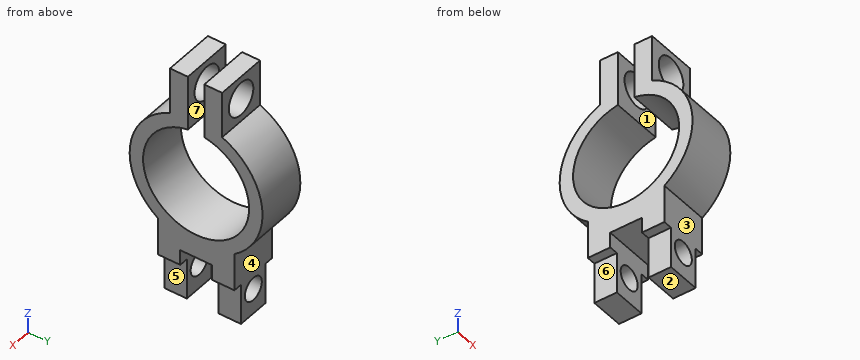
```python
from build123d import *

# Parameters (mm, degrees)
PAD_DEPTH       = 10
POCKET_DEPTH    = 10
SKETCH004_R     = 3.25
POCKET002_DEPTH = 15
SKETCH005_R     = 2.25
POCKET003_DEPTH = 15
SKETCH006_W     = 8
SKETCH006_H     = 1.75
POCKET004_DEPTH = 15


with BuildPart() as part:
    # Sketch → Pad (new body)
    with BuildSketch(Plane.YZ):
        with BuildLine():
            ThreePointArc((-1.6, 10.250884), (0, -10.375), (1.6, 10.250884))
            Line((1.6, 20.997843), (1.6, 10.250884))
            Line((1.6, 20.997843), (5.1, 20.997843))
            Line((5.1, 20.997843), (5.1, 11.957843))
            ThreePointArc((7.5, -10.61838), (12.92716, 1.374242), (5.1, 11.957843))
            Line((7.5, -25.99838), (7.5, -10.61838))
            Line((-7.5, -25.99838), (7.5, -25.99838))
            Line((-7.5, -25.99838), (-7.5, -10.61838))
            ThreePointArc((-5.1, 11.957843), (-12.92716, 1.374242), (-7.5, -10.61838))
            Line((-5.1, 20.997843), (-5.1, 11.957843))
            Line((-1.6, 20.997843), (-5.1, 20.997843))
            Line((-1.6, 20.997843), (-1.6, 10.250884))
        make_face()
    extrude(amount=PAD_DEPTH)

    # Sketch003 → Pocket (cut)
    with BuildSketch(Plane(origin=(0, 0, 0), x_dir=(0, 1, 0), z_dir=(-1, 0, 0))):
        Polygon((0, 25.99838), (-3.1, 25.99838), (-3.1, 14.99838), (0, 14.99838), (3.1, 14.99838), (3.1, 25.99838), align=None)
    extrude(amount=-POCKET_DEPTH, mode=Mode.SUBTRACT)

    # Sketch004 (on Face9 of Pocket) → Pocket002 (cut)
    with BuildSketch(Plane.ZX.offset(5.1)):
        with Locations((16.507843, 5)):
            Circle(SKETCH004_R)
    extrude(amount=-POCKET002_DEPTH, mode=Mode.SUBTRACT)

    # Sketch005 (on Face12 of Pocket002) → Pocket003 (cut)
    with BuildSketch(Plane.ZX.offset(7.5)):
        with Locations((-20.99838, 5)):
            Circle(SKETCH005_R)
    extrude(amount=-POCKET003_DEPTH, mode=Mode.SUBTRACT)

    # Sketch006 (on Face12 of Pocket003) → Pocket004 (cut)
    with BuildSketch(Plane.ZX.offset(7.5)):
        with Locations((-21.99838, 9.125)):
            Rectangle(SKETCH006_W, SKETCH006_H)
        with Locations((-21.99838, 0.875)):
            Rectangle(SKETCH006_W, SKETCH006_H)
    extrude(amount=-POCKET004_DEPTH, mode=Mode.SUBTRACT)


solid = part.part
```
The model under review builds one solid part; all positions refer to its coordinate system, in mm. Face numbers are marked on the shaded views. A direction names the side the tool comes from. Round coordinates to 2 decimals unless told otherwise and drop trailing zeros. Loops run counter-clockwise (first coordinate to the right, second up) from the corner with the lowest first, then second, coordinate; pieces in that order, holes last. Notation, with made-up numbers: M 46,-23 L 86,-23 A14 cw 86,4 Z; hole C 0.25,40 d8. An arc over 180 degrees is marked long. Write item = value, one per line.
Item 1: For line 1 (Y direction, x = 6.75, z = 0) (3 decimals); line 2 (Z direction, x = 6, y = 3.5); line 3 (Y direction, x = 2.5, z = -22), list the stretches that pass through material, from the lowest coordinate up. Write a range as [from, to].
Return value:
line_1 = [-13, -10.375], [10.375, 13]
line_2 = [-26, -23.01], [-18.98, -9.77], [9.77, 13.42], [19.6, 21]
line_3 = [-7.5, -3.1], [3.1, 7.5]
Item 2: Machinability: for the marked faces 5, 6 and 7, which of the approach directions +Z, -Z, +X, -X, +Y, -Y give a long, thin tool a straight path to every point of the face, cutting with its end or side? Answer none if there is none.
Return value:
face_5 = -Z, +X, +Y, -Y
face_6 = -Z, -X, +Y, -Y
face_7 = +Z, +X, -X
Item 3: Take a section at A-A on x = 5. State how many separate pieces and enclosed holes the cut face has, then the cut area to 3 significant figures.
Return value:
separate_pieces = 5
enclosed_holes = 0
area = 297 mm2
Item 4: Take a section at D-D on y = -4. Write out the cut boundary in (x, z).
Return value:
outline = M 0,-18 L 1.75,-18 L 1.75,-26 L 8.25,-26 L 8.25,-18 L 10,-18 L 10,-9.57 L 0,-9.57 Z; M 0,9.57 L 10,9.57 L 10,21 L 0,21 Z; hole C 5,16.51 d6.5; hole C 5,-21 d4.5
Item 5: The part is to be moulded in two halves that separate along Y. For the marked faces 1, 2, 3 and 4, say which applies: released by +Y, released by -Y, zero draft, split by the parting line, or undercut.
Return value:
face_1 = undercut
face_2 = zero draft
face_3 = released by -Y
face_4 = released by +Y
Item 6: Take a section at C-C on y = 8. Write out the cut boundary in (x, z), then the cut area to 3 significant figures.
Return value:
outline = M 0,-10.25 L 10,-10.25 L 10,-6.61 L 0,-6.61 Z; M 0,6.61 L 10,6.61 L 10,10.25 L 0,10.25 Z
area = 72.8 mm2
Item 7: Insertion check: P1, Ø5, axis at x = 6.5, y = 0, coming from the -Z side; P2, Ø5, axis at x = 3.5, z = -15, coming from the -Y side; P3, Ø2.5, axis at x = 5, z = -21, coming from the +Y side; P4, Ø3, axis at x = 4.5, z = 3.5, coming from the -Y side. Each pin has a flat end and moves straight along its axis. Give the tip position at first contact, or say it passes through.
Return value:
P1 = -15
P2 = -7.5
P3 = through
P4 = -12.85
Item 8: Take a section at B-B on z = 0. Write out the cut boundary in (x, y) (3 decimals), then the cut area to 3 significant figures.
Return value:
outline = M 0,-13 L 10,-13 L 10,-10.375 L 0,-10.375 Z; M 0,10.375 L 10,10.375 L 10,13 L 0,13 Z
area = 52.5 mm2
